Could you check a few things on this drawing? It's one solid part, dimensions in mm from its lowest x, y, z. Give positions to 0.01 mm unless a question says otherwise; leave off trailing zeros. Order: outer loops, then holes, each group sorted by start corner. A loop starts at its lowest first (then second) coordinate and runs counter-clockwise, first axis right, second up.
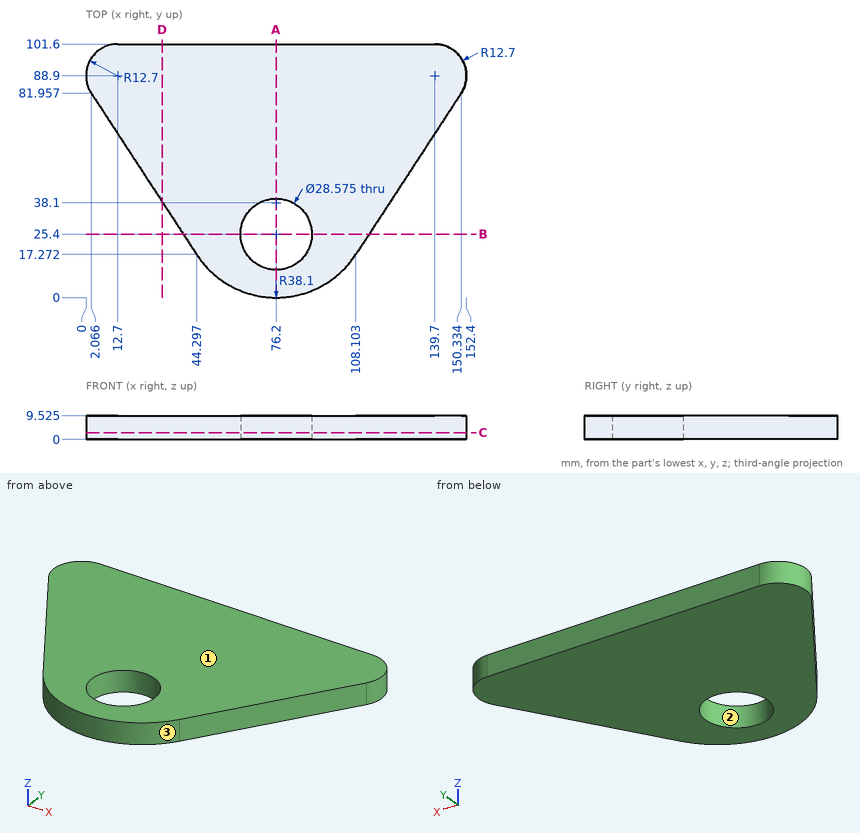
1) If I drill on line 1 (Y direction, x = 76.2, z = 3.75); line 2 (Y direction, x = 86.5, z = 2.5); line 3 (X direction, y = 19.5, z = 1.25), over which ranges is the centre line in solid material (lowest first)?
2) Suppose I cut it at A-A (x = 76.2). Please give me the cut outline in (y, z) (1 decimal).
3) We'd pull the mould along X, two halves only. Please class the marked faces 1, 2 and 3: +X half, -X half, draft (parallel to the pull), parting line (faces both ways), or undercut.
4) I'm going to push flat-ended pins straight in: pin 1 Ø1 at (x, z) = (71.5, 3) entering from -Y; pin 2 Ø1 at (y, z) = (26, 6) entering from -X; pin 3 Ø1.5 at (y, z) = (41.5, 7.5) entering from +X. Where does each tip first touch, or does it pass through?
5) Suppose I cut it at C-C (z = 2.75). Please give me the cut outline in (x, y) (1 decimal).
6) Suppose I cut it at B-B (y = 25.4). Please give me the cut outline in (x, z) (1 decimal), and give its area (3 significant figures).
7) Suppose I cut it at D-D (x = 30.5). Please give me the cut outline in (y, z) (1 decimal), and give its area (3 significant figures).
Results:
1. line 1: y = 0 to 11.11, 39.69 to 101.6
1. line 2: y = 1.42 to 15.5, 35.3 to 101.6
1. line 3: x = 42.84 to 63.19, 89.21 to 109.56
2. outline: (0, 0) - (11.1, 0) - (11.1, 9.5) - (0, 9.5) - close; (39.7, 0) - (101.6, 0) - (101.6, 9.5) - (39.7, 9.5) - close
3. face 1: draft
3. face 2: undercut
3. face 3: parting line
4. pin 1: stops at y = 0.23
4. pin 2: stops at x = 38.27
4. pin 3: stops at x = 124.41
5. outline: (2.1, 82) - (44.3, 17.3) arc R38.1 ccw to (108.1, 17.3) - (150.3, 82) arc R12.7 ccw to (139.7, 101.6) - (12.7, 101.6) arc R12.7 ccw to start; hole circle Ø28.6 at (76.2, 25.4)
6. outline: (39, 0) - (61.9, 0) - (61.9, 9.5) - (39, 9.5) - close; (90.5, 0) - (113.4, 0) - (113.4, 9.5) - (90.5, 9.5) - close
6. area: 437 mm2
7. outline: (38.4, 0) - (101.6, 0) - (101.6, 9.5) - (38.4, 9.5) - close
7. area: 602 mm2
